Read the model definition and answer for the solid it produces. Units are mm, in the model's axes. A direction names the side the tool comes from. Give positions to 0.01 mm unless a question says otherwise; leave off trailing zeros. Order: outer loops, then holes, each group sorted by start corner. A loop starts at its lowest first (then second) coordinate and runs counter-clockwise, first axis right, second up. Notation, with made-up numbers: (43, -2) - (61, -2) arc R22 cw to (61, 31) - close; hole circle Ø3 at (34, 11). An arc over 180 degrees is marked (long way). Return JSON: item names as keys, results as strings.
```python
from build123d import *

# Parameters (mm, degrees)
SKETCH_1_R          = 7
EXTRUDE_1_DEPTH     = 4
SKETCH_2_R          = 7
SKETCH_2_R_2        = 4.5
EXTRUDE_2_DEPTH     = 2.5
SKETCH_3_R          = 1
CUT_EXTRUDE_1_DEPTH = 2.5
CUT_EXTRUDE_2_DEPTH = 2
SKETCH_5_R          = 18
SKETCH_5_R_2        = 7
EXTRUDE_3_DEPTH     = 2.5
EXTRUDE_4_DEPTH     = 2


with BuildPart() as part:
    # 草图1 → 凸台-拉伸1 (new body)
    with BuildSketch(Plane(origin=(0, 0, 0), x_dir=(1, 0, 0), z_dir=(0, 1, 0))):
        with Locations(Location((0, 0, 0), (0, 0, 270))):
            Circle(SKETCH_1_R)
    extrude(amount=EXTRUDE_1_DEPTH)

    # 草图2 → 凸台-拉伸2 (add)
    with BuildSketch(Plane(origin=(0, 4, 0), x_dir=(1, 0, 0), z_dir=(0, 1, 0))):
        with Locations(Location((0, 0, 0), (0, 0, 270))):
            Circle(SKETCH_2_R)
        with Locations(Location((0, 0, 0), (0, 0, 270))):
            Circle(SKETCH_2_R_2, mode=Mode.SUBTRACT)
    extrude(amount=EXTRUDE_2_DEPTH)

    # 草图3 → 切除-拉伸1 (cut)
    with BuildSketch(Plane(origin=(0, 4, 0), x_dir=(1, 0, 0), z_dir=(0, 1, 0))):
        with Locations(Location((0, 0, 0), (0, 0, 270))):
            Circle(SKETCH_3_R)
    extrude(amount=-CUT_EXTRUDE_1_DEPTH, mode=Mode.SUBTRACT)

    # 草图4 → 切除-拉伸2 (cut)
    with BuildSketch(Plane.XZ):
        Polygon((1.459083967, -2.490864772), (2.886694153, 0.018171396), (1.427610186, 2.509036167), (-1.459083967, 2.490864772), (-2.886694153, -0.018171396), (-1.427610186, -2.509036167), align=None)
    extrude(amount=-CUT_EXTRUDE_2_DEPTH, mode=Mode.SUBTRACT)

    # 草图5 → 凸台-拉伸3 (add)
    with BuildSketch(Plane(origin=(0, 2, 0), x_dir=(1, 0, 0), z_dir=(0, 1, 0))):
        with Locations(Location((0, 0, 0), (0, 0, 270))):
            Circle(SKETCH_5_R)
        with Locations(Location((0, 0, 0), (0, 0, 270))):
            Circle(SKETCH_5_R_2, mode=Mode.SUBTRACT)
    extrude(amount=EXTRUDE_3_DEPTH)

    # 草图6 → 凸台-拉伸4 (add, symmetric)
    with BuildSketch(Plane(origin=(7, 0, 0), x_dir=(0, 0, -1), z_dir=(1, 0, 0))):
        with BuildLine():
            Line((-6.459228818, 2), (-0.994639994, -11.532205447))
            ThreePointArc((-0.994639994, -11.532205447), (3.965427991, -14.168883056), (7.420905758, -9.740111597))
            Line((7.420905758, -9.740111597), (7, 2))
            Line((7, 2), (-6.459228818, 2))
        make_face()
        Polygon((4.232968046, -7.260851368), (1.361669462, -7.559142793), (0.184348122, -10.194906021), (1.878325366, -12.532377824), (4.74962395, -12.234086399), (5.92694529, -9.598323171), align=None, mode=Mode.SUBTRACT)
    extrude_4 = extrude(amount=EXTRUDE_4_DEPTH, both=True)

    # 镜向1: 凸台-拉伸4 across plane
    add(extrude_4.mirror(Plane(origin=(0, 0, 0), x_dir=(0, 0, 1), z_dir=(1, 0, 0))))


solid = part.part
```
Q1. A cutting plane is placed at D-D (x = 5.5). Write down the section's boundary in (y, z).
Values:
{"outline": "(-11.53, 0.99) arc R4.37 ccw to (-9.74, -7.42) - (2, -7) - (2, -17.14) - (4.5, -17.14) - (4.5, -4.33) - (6.5, -4.33) - (6.5, 4.33) - (4.5, 4.33) - (4.5, 17.14) - (2, 17.14) - (2, 6.46) - close; hole (-12.53, -1.88) - (-12.23, -4.75) - (-9.6, -5.93) - (-7.26, -4.23) - (-7.56, -1.36) - (-10.19, -0.18) - close"}
Q2. A cutting plane is placed at A-A (y = -4.5). Write down the section's boundary in (x, z).
Values:
{"outline": "(-9, -7.23) - (-5, -7.23) - (-5, 3.83) - (-9, 3.83) - close; (5, -7.23) - (9, -7.23) - (9, 3.83) - (5, 3.83) - close"}
Q3. Consider L1, parallel to X at y = -7.5, z = -5; L2, parallel to X at y = 4.85, z = 0; L3, parallel to Y at x = -11, z = -7.5. Determine where each line is inside the solid, lowest interval first.
Values:
{"L1": "x = -9 to -5, 5 to 9", "L2": "x = -7 to -4.5, 4.5 to 7", "L3": "y = 2 to 4.5"}
Q4. Determine the mould class of faces 1 (the flat face through (2.163, 0.986, -1.254)), 2 (the flat face through (-1, 4, 1)), 3 (the flat face through (-2.2, 0, 1.5)), 4 (the flat face through (-7.03, -10.93, -5.33)) for opening direction Y: released by +Y, released by -Y, zero draft, split by the parting line, or undercut.
Values:
{"face 1": "zero draft", "face 2": "released by +Y", "face 3": "released by -Y", "face 4": "undercut"}
Q5. For faces 5 (the cylindrical face through (-6.834, 5.486, -1.517)), 6 (the flat face through (-2.167, 0.986, -1.246)), 7 (the flat face through (7.03, -10.93, -5.33)), 8 (the flat face through (9, -4, -2)), determine the directions among +Z, -Z, +X, -X, +Y, -Y from which every point of the face is accessible in a straight line to the end or side of a thin tool.
Values:
{"face 5": "+Y", "face 6": "-Y", "face 7": "+X, -X", "face 8": "+Z, -Z, +X, -Y"}
Q6. A cutting plane is placed at B-B (z = -3.5). Write down the section's boundary in (x, y), and give its area (3 significant figures).
Values:
{"outline": "(-17.66, 2) - (-9, 2) - (-9, -7.34) - (-5, -7.34) - (-5, 0) - (5, 0) - (5, -7.34) - (9, -7.34) - (9, 2) - (17.66, 2) - (17.66, 4.5) - (6.06, 4.5) - (6.06, 6.5) - (2.83, 6.5) - (2.83, 4) - (-2.83, 4) - (-2.83, 6.5) - (-6.06, 6.5) - (-6.06, 4.5) - (-17.66, 4.5) - close; (-9, -14.24) - (-5, -14.24) - (-5, -12.36) - (-9, -12.36) - close; (5, -14.24) - (9, -14.24) - (9, -12.36) - (5, -12.36) - close", "area": "208 mm²"}
Q7. A cutting plane is placed at C-C (x = 0). Write down the section's boundary in (y, z).
Values:
{"outline": "(0, -7) - (2, -7) - (2, -18) - (4.5, -18) - (4.5, -7) - (6.5, -7) - (6.5, -4.5) - (4, -4.5) - (4, -1) - (2, -1) - (2, -2.5) - (0, -2.5) - close; (0, 2.5) - (2, 2.5) - (2, 1) - (4, 1) - (4, 4.5) - (6.5, 4.5) - (6.5, 7) - (4.5, 7) - (4.5, 18) - (2, 18) - (2, 7) - (0, 7) - close"}
Q8. Given pin 1 (3 mm diameter, centred on x = 2.5, z = 14, fed in from -Y); pin 2 (4 mm diameter, centred on y = -2.5, z = 1.5, fed in from +X); pin 3 (8 mm diameter, centred on x = 8, y = -11, fed in from +Z); pin 4 (12 mm diameter, centred on x = 6, z = 10, fed in from +Y), each flat-ended and moving along its own axis, determine where each tip first touches the part or whether it passes through.
Values:
{"pin 1": "stops at y = 2", "pin 2": "stops at x = 9", "pin 3": "stops at z = 2.82", "pin 4": "stops at y = 6.5"}
